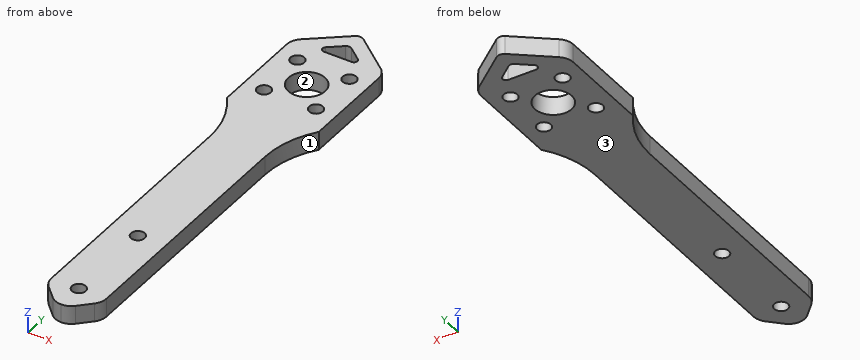
```python
from build123d import *

# Parameters (mm, degrees)
F0_R     = 1.5
F0_R_2   = 4
F1_DEPTH = 4


with BuildPart() as f1:
    # F0 (on Top) → F1 (new body)
    with BuildSketch(Plane.XY):
        with BuildLine():
            Line((6, -77.216061), (6, -23.5))
            ThreePointArc((6, -23.5), (7.026334, -17.175445), (10, -11.5))
            Line((10, -11.5), (10, 8.817813))
            ThreePointArc((10, 8.817813), (9.654561, 10.333974), (8.686433, 11.550854))
            Line((8.686433, 11.550854), (0.937043, 17.750366))
            ThreePointArc((0.937043, 17.750366), (0, 18.079063), (-0.937043, 17.750366))
            Line((-0.937043, 17.750366), (-8.686433, 11.550854))
            ThreePointArc((-8.686433, 11.550854), (-9.654561, 10.333974), (-10, 8.817813))
            Line((-10, 8.817813), (-10, -11.5))
            ThreePointArc((-10, -11.5), (-7.026334, -17.175445), (-6, -23.5))
            Line((-6, -23.5), (-6, -77.216061))
            ThreePointArc((-6, -77.216061), (-5.733578, -78.555453), (-4.974874, -79.690934))
            Line((-4.974874, -79.690934), (-2.474874, -82.190934))
            ThreePointArc((-2.474874, -82.190934), (-1.339392, -82.949639), (0, -83.216061))
            ThreePointArc((0, -83.216061), (1.339392, -82.949639), (2.474874, -82.190934))
            Line((2.474874, -82.190934), (4.974874, -79.690934))
            ThreePointArc((4.974874, -79.690934), (5.733578, -78.555453), (6, -77.216061))
        make_face()
        with Locations((0, -77.216061)):
            Circle(F0_R, mode=Mode.SUBTRACT)
        with Locations((0, -57.216061)):
            Circle(F0_R, mode=Mode.SUBTRACT)
        with Locations((-5.656854, -5.656854)):
            Circle(F0_R, mode=Mode.SUBTRACT)
        with Locations((-5.656854, 5.656854)):
            Circle(F0_R, mode=Mode.SUBTRACT)
        Circle(F0_R_2, mode=Mode.SUBTRACT)
        with BuildLine():
            Line((3.059571, 10.5), (0, 10.5))
            Line((0, 10.5), (-3.059571, 10.5))
            ThreePointArc((-3.059571, 10.5), (-3.767292, 11.001745), (-3.528092, 11.835652))
            Line((-3.528092, 11.835652), (-0.624695, 14.158369))
            ThreePointArc((-0.624695, 14.158369), (0, 14.377501), (0.624695, 14.158369))
            Line((0.624695, 14.158369), (3.528092, 11.835652))
            ThreePointArc((3.528092, 11.835652), (3.767292, 11.001745), (3.059571, 10.5))
        make_face(mode=Mode.SUBTRACT)
        with Locations((5.656854, -5.656854)):
            Circle(F0_R, mode=Mode.SUBTRACT)
        with Locations((5.656854, 5.656854)):
            Circle(F0_R, mode=Mode.SUBTRACT)
    extrude(amount=F1_DEPTH)


solid = f1.part
```
The model under review builds one solid part; all positions refer to its coordinate system, in mm. Face numbers are marked on the shaded views. Round coordinates to 2 decimals unless told otherwise and drop trailing zeros. Loops run counter-clockwise (first coordinate to the right, second up) from the corner with the lowest first, then second, coordinate; pieces in that order, holes last.
1) The part is to be moulded in two halves that separate along Y. For the marked faces 1, 2 and 3, say which applies: pulls with the +Y half, pulls with the -Y half, needs draft (parallel to the pull), parting line crosses it, or undercut.
Values follow:
face 1: pulls with the -Y half
face 2: undercut
face 3: needs draft
2) Wall thickness on line 1 along Y through (x, z) = (0, 3.25); line 2 along Y through (x, z) = (3.5, 1.15); line 3 along Y through (x, z) = (3.25, 2.65): over which ranges is each line inside the solid? List them lowest first.
Values follow:
line 1: y = -83.22 to -78.72, -75.72 to -58.72, -55.72 to -4, 4 to 10.5, 14.38 to 18.08
line 2: y = -81.17 to -1.94, 1.94 to 10.64, 11.86 to 15.7
line 3: y = -81.42 to -2.33, 2.33 to 10.52, 12.06 to 15.9
3) Clearance check with flat-ended pins moving along their axes: P1, Ø2.5, axis at x = -5.66, y = 5.66, coming from the +Z side; P2, Ø1.5, axis at x = 1.5, y = -10.5, coming from the -Z side; P3, Ø2, axis at y = -47, z = 2, coming from the -X side; P4, Ø1, axis at x = -6, z = 1.5, coming from the +Y side. State where each tip first meets the part, or that it passes through.
Values follow:
P1: passes through
P2: stops at z = 0
P3: stops at x = -6
P4: stops at y = 14.1
4) Consider section C-C on y = -49.5. State the section outline as (x, z) points, then the cut area to 3 significant figures.
Values follow:
outline: (-6, 0) - (6, 0) - (6, 4) - (-6, 4) - close
area: 48.0 mm2
5) Consider section A-A on y = 0. State the section outline as (x, z) points.
Values follow:
outline: (-10, 0) - (-4, 0) - (-4, 4) - (-10, 4) - close; (4, 0) - (10, 0) - (10, 4) - (4, 4) - close
6) Consider section B-B on z = 1.55. Give the number of separate pieces and of enclosed holes in the cut face, then the cut area to 3 significant figures.
Values follow:
separate pieces: 1
enclosed holes: 8
area: 1,280 mm2
